For this review, take the finished solid that the model builds, in its own axes (mm). A direction names the side the tool comes from. Coordinates: 2 decimals unless noted, no trailing zeros. Order: outer loops, then holes, each group sorted by start corner. A loop starts at its lowest first (then second) coordinate and runs counter-clockwise, first axis right, second up. Notation, with made-up numbers: M 48,-17.75 L 66,-17.75 A22 ccw 66,-11.75 Z; hole C 76.5,-28.5 d11. An arc over 180 degrees is marked long. Use CSV: the item, a comma, the result in double quotes.
```python
from build123d import *

# Parameters (mm, degrees)
ESTRUSIONE_ESTRUSIONE1_DEPTH = 225
TAGLIO_ESTRUSIONE1_DEPTH     = 90
SVUOTA1_T                    = -15
TAGLIO_ESTRUSIONE2_START     = -20
SCHIZZO4_R                   = 40
TAGLIO_ESTRUSIONE2_DEPTH     = 20
ESTRUSIONE_ESTRUSIONE2_START = 10
SCHIZZO6_W                   = 154.725791786
SCHIZZO6_H                   = 435
SCHIZZO6_R                   = 40
ESTRUSIONE_ESTRUSIONE2_DEPTH = 10
ESTRUSIONE_ESTRUSIONE3_DEPTH = 15
TAGLIO_ESTRUSIONE12_DEPTH    = 491.866580651
TAGLIO_ESTRUSIONE13_DEPTH    = 20


with BuildPart() as part:
    # Schizzo1 → Estrusione-Estrusione1 (new, symmetric)
    with BuildSketch(Plane.XY):
        Polygon((-125, 0), (125, 0), (125, 25), (60, 190), (-60, 190), (-125, 25), align=None)
    extrude(amount=ESTRUSIONE_ESTRUSIONE1_DEPTH, both=True)

    # Schizzo2 → Taglio-Estrusione1 (cut)
    with BuildSketch(Plane(origin=(0, 190, 0), x_dir=(1, 0, 0), z_dir=(0, 1, 0))):
        with BuildLine():
            ThreePointArc((0, -110), (-25, -135), (0, -160))
            Line((0, -160), (0, -135))
            Line((0, -135), (0, -110))
        make_face()
        with BuildLine():
            Line((0, -135), (0, -160))
            ThreePointArc((0, -160), (17.67766953, -152.67766953), (25, -135))
            ThreePointArc((25, -135), (17.67766953, -117.32233047), (0, -110))
            Line((0, -110), (0, -135))
        make_face()
        with BuildLine():
            ThreePointArc((0, -20), (-25, -45), (0, -70))
            Line((0, -70), (0, -45))
            Line((0, -45), (0, -20))
        make_face()
        with BuildLine():
            Line((0, -45), (0, -70))
            ThreePointArc((0, -70), (17.67766953, -62.67766953), (25, -45))
            ThreePointArc((25, -45), (17.67766953, -27.32233047), (0, -20))
            Line((0, -20), (0, -45))
        make_face()
        with BuildLine():
            ThreePointArc((0, 70), (-25, 45), (0, 20))
            Line((0, 20), (0, 45))
            Line((0, 45), (0, 70))
        make_face()
        with BuildLine():
            Line((0, 45), (0, 20))
            ThreePointArc((0, 20), (17.67766953, 27.32233047), (25, 45))
            ThreePointArc((25, 45), (17.67766953, 62.67766953), (0, 70))
            Line((0, 70), (0, 45))
        make_face()
        with BuildLine():
            ThreePointArc((0, 160), (-25, 135), (0, 110))
            Line((0, 110), (0, 135))
            Line((0, 135), (0, 160))
        make_face()
        with BuildLine():
            Line((0, 135), (0, 110))
            ThreePointArc((0, 110), (17.67766953, 117.32233047), (25, 135))
            ThreePointArc((25, 135), (17.67766953, 152.67766953), (0, 160))
            Line((0, 160), (0, 135))
        make_face()
    extrude(amount=-TAGLIO_ESTRUSIONE1_DEPTH, mode=Mode.SUBTRACT)

    # Svuota1
    svuota1_openings = [part.faces().sort_by_distance(p)[0] for p in [
        (0, 83.334466349, 225),
    ]]
    offset(amount=SVUOTA1_T, openings=svuota1_openings, kind=Kind.INTERSECTION)

    # Schizzo4 → Taglio-Estrusione2 (cut)
    with BuildSketch(Plane.XZ.offset(-85).offset(TAGLIO_ESTRUSIONE2_START)):
        with Locations(Location((0, -135, 0), (0, 0, 90))):
            Circle(SCHIZZO4_R)
        with Locations(Location((0, -45, 0), (0, 0, 90))):
            Circle(SCHIZZO4_R)
        with Locations(Location((0, 45, 0), (0, 0, 90))):
            Circle(SCHIZZO4_R)
        with Locations(Location((0, 135, 0), (0, 0, 90))):
            Circle(SCHIZZO4_R)
    extrude(amount=TAGLIO_ESTRUSIONE2_DEPTH, mode=Mode.SUBTRACT)

    # Schizzo6 → Estrusione-Estrusione2 (add)
    with BuildSketch(Plane(origin=(0, 105, 0), x_dir=(1, 0, 0), z_dir=(0, 1, 0)).offset(ESTRUSIONE_ESTRUSIONE2_START)):
        with Locations((0, -7.5)):
            Rectangle(SCHIZZO6_W, SCHIZZO6_H)
        with Locations(Location((0, 135, 0), (0, 0, 270))):
            Circle(SCHIZZO6_R, mode=Mode.SUBTRACT)
        with Locations(Location((0, 45, 0), (0, 0, 270))):
            Circle(SCHIZZO6_R, mode=Mode.SUBTRACT)
        with Locations(Location((0, -45, 0), (0, 0, 270))):
            Circle(SCHIZZO6_R, mode=Mode.SUBTRACT)
        with Locations(Location((0, -135, 0), (0, 0, 270))):
            Circle(SCHIZZO6_R, mode=Mode.SUBTRACT)
    extrude(amount=-ESTRUSIONE_ESTRUSIONE2_DEPTH)

    # Schizzo7 → Estrusione-Estrusione3 (add)
    with BuildSketch(Plane.XY.offset(225)):
        Polygon((-125, 25), (-125, 0), (125, 0), (125, 25), (60, 190), (-60, 190), align=None)
    extrude(amount=-ESTRUSIONE_ESTRUSIONE3_DEPTH)

    # Schizzo12 → Taglio-Estrusione12 (cut, through all)
    with BuildSketch(Plane.XY.offset(-210)):
        with BuildLine():
            ThreePointArc((35, 60), (24.748737342, 84.748737342), (0, 95))
            Line((0, 95), (0, 25))
            ThreePointArc((0, 25), (24.748737342, 35.251262658), (35, 60))
        make_face()
        with BuildLine():
            Line((0, 25), (0, 95))
            ThreePointArc((0, 95), (-35, 60), (0, 25))
        make_face()
    extrude(amount=-TAGLIO_ESTRUSIONE12_DEPTH, mode=Mode.SUBTRACT)

    # Schizzo13 → Taglio-Estrusione13 (cut)
    with BuildSketch(Plane(origin=(0, 190, 0), x_dir=(1, 0, 0), z_dir=(0, 1, 0))):
        with BuildLine():
            Line((0, 97.5), (0, 95))
            ThreePointArc((0, 95), (-15.307337295, 98.0448187), (-28.284271247, 106.715728753))
            Line((-28.284271247, 106.715728753), (-26.516504294, 108.483495706))
            ThreePointArc((-26.516504294, 108.483495706), (-14.350628714, 100.354517531), (0, 97.5))
        make_face()
        with BuildLine():
            Line((26.516504294, 161.516504294), (28.284271247, 163.284271247))
            ThreePointArc((28.284271247, 163.284271247), (15.307337295, 171.9551813), (0, 175))
            Line((0, 175), (0, 172.5))
            ThreePointArc((0, 172.5), (14.350628714, 169.645482469), (26.516504294, 161.516504294))
        make_face()
        with BuildLine():
            Line((-26.516504294, 18.483495706), (-28.284271247, 16.715728753))
            ThreePointArc((-28.284271247, 16.715728753), (-15.307337295, 8.0448187), (0, 5))
            Line((0, 5), (0, 7.5))
            ThreePointArc((0, 7.5), (-14.350628714, 10.354517531), (-26.516504294, 18.483495706))
        make_face()
        with BuildLine():
            Line((26.516504294, 71.516504294), (28.284271247, 73.284271247))
            ThreePointArc((28.284271247, 73.284271247), (15.307337295, 81.9551813), (0, 85))
            Line((0, 85), (0, 82.5))
            ThreePointArc((0, 82.5), (14.350628714, 79.645482469), (26.516504294, 71.516504294))
        make_face()
        with BuildLine():
            Line((-26.516504294, -71.516504294), (-28.284271247, -73.284271247))
            ThreePointArc((-28.284271247, -73.284271247), (-15.307337295, -81.9551813), (0, -85))
            Line((0, -85), (0, -82.5))
            ThreePointArc((0, -82.5), (-14.350628714, -79.645482469), (-26.516504294, -71.516504294))
        make_face()
        with BuildLine():
            Line((26.516504294, -18.483495706), (28.284271247, -16.715728753))
            ThreePointArc((28.284271247, -16.715728753), (15.307337295, -8.0448187), (0, -5))
            Line((0, -5), (0, -7.5))
            ThreePointArc((0, -7.5), (14.350628714, -10.354517531), (26.516504294, -18.483495706))
        make_face()
        with BuildLine():
            Line((-26.516504294, -161.516504294), (-28.284271247, -163.284271247))
            ThreePointArc((-28.284271247, -163.284271247), (-15.307337295, -171.9551813), (0, -175))
            Line((0, -175), (0, -172.5))
            ThreePointArc((0, -172.5), (-14.350628714, -169.645482469), (-26.516504294, -161.516504294))
        make_face()
        with BuildLine():
            Line((26.516504294, -108.483495706), (28.284271247, -106.715728753))
            ThreePointArc((28.284271247, -106.715728753), (15.307337295, -98.0448187), (0, -95))
            Line((0, -95), (0, -97.5))
            ThreePointArc((0, -97.5), (14.350628714, -100.354517531), (26.516504294, -108.483495706))
        make_face()
    extrude(amount=-TAGLIO_ESTRUSIONE13_DEPTH, mode=Mode.SUBTRACT)


solid = part.part
```
Item 1: For faces 1 (the face through (-1, 145, 210)), 2 (the face through (-15.1, 182.6, -97.96)), 3 (the face through (-125, 13, 3)), list the 3-axis set-ups (+Z, -Z, +X, -X, +Y, -Y) from which the entire face can be reached by the end or side of a thin tool; tool diameter is ignored.
Solutions:
face 1,"none"
face 2,"+Y"
face 3,"+Z, -Z, -X, +Y, -Y"
Item 2: To check wall thickness, follow line 1 along Z through (x, y) = (90.5, 37.5); line 2 along X through (y, z) = (21.5, 10); line 3 along X through (y, z) = (166, 63). State the ranges of each line that lie inside material, in increasing order. Write a range as [from, to].
Solutions:
line 1,"[-225, -210], [210, 225]"
line 2,"[-125, -110], [110, 125]"
line 3,"[-69.45, -53.33], [-35.72, -17.35], [17.35, 35.72], [53.33, 69.45]"
Item 3: Draft analysis for pull direction Y (two halves, no side actions). For faces 4 (the face through (-2, 0, 3)), 5 (the face through (-2, 61, 210)), 6 (the face through (-14.541, 180.14, -100.434)), state which applies: released by +Y, released by -Y, zero draft, split by the parting line, or undercut.
Solutions:
face 4,"released by -Y"
face 5,"undercut"
face 6,"zero draft"
Item 4: Add section D-D on y = 44.5. State the section outline as (x, z) points.
Solutions:
outline,"M -117.32,-225 L -31.38,-225 L -31.38,-210 L -101.2,-210 L -101.2,210 L 101.2,210 L 101.2,-210 L 31.38,-210 L 31.38,-225 L 117.32,-225 L 117.32,225 L -117.32,225 Z"
Item 5: Add section A-A on z = 180. State the section outline as (x, y) points, and give its area (3 significant figures).
Solutions:
outline,"M -125,0 L 125,0 L 125,25 L 60,190 L -60,190 L -125,25 Z; hole M -110,15 L 110,15 L 110,22.15 L 77.36,105 L -77.36,105 L -110,22.15 Z; hole M -73.42,115 L 73.42,115 L 49.79,175 L -49.79,175 Z"
area,"12,300 mm^2"
Item 6: Add section B-B on y = 151.5. State how many separate pieces and enclosed holes the cut face has, and give its area (3 significant figures).
Solutions:
separate pieces,"5"
enclosed holes,"5"
area,"30,300 mm^2"
Item 7: Add section C-C on x = 66. State the section outline as (y, z) points.
Solutions:
outline,"M 0,-225 L 174.77,-225 L 174.77,225 L 0,225 Z; hole M 15,-210 L 105,-210 L 105,210 L 15,210 Z; hole M 115,-210 L 133.84,-210 L 133.84,210 L 115,210 Z"
Item 8: Clearance check with flat-ended pins moving along their axes: pin 1 Ø0.8 at (y, z) = (181.5, -96) entering from -X; pin 2 Ø1.2 at (y, z) = (179.5, 83.5) entering from -X; pin 3 Ø10 at (y, z) = (84, 25) entering from -X. State where each tip first meets the part, or that it passes through.
Solutions:
pin 1,"x = -63.51"
pin 2,"x = -64.37"
pin 3,"x = -103.73"
